Verification items for the finished model (mm, model axes). Face numbers are marked on the shaded views. A direction names the side the tool comes from. Coordinates: 2 decimals unless noted, no trailing zeros. Order: outer loops, then holes, each group sorted by start corner. A loop starts at its lowest first (then second) coordinate and runs counter-clockwise, first axis right, second up. Notation, with made-up numbers: M -35,6 L -1,6 A19 ccw -1,26 Z; hole C 89.5,29.25 d11. An arc over 180 degrees is marked long. Answer as a JSON object with one key per item and string values. Group by question number.
(1) Cross-section at C-C (y = -298). Enter the section's corners in (x, z).
(2) Cross-section at A-A (x = 70). Enter the section's corners in (y, z).
(3) Access from +Z, -Z, +X, -X, +Y, -Y to the whole of each face (thin tool, end or side, straight path). Record for the marked faces 1 and 2.
(4) Cross-section at B-B (z = 962). Enter the section's corners in (x, y), plus the area to 3 significant figures.
(5) Material ranges on line 1 (Y direction, x = 101, z = 986); line 2 (X direction, y = -295, z = 1023); line 3 (Z direction, x = 77.5, y = -305.5), recorded low to high.
(6) Cross-section at D-D (x = 33.5). Enter the section's corners in (y, z).
(7) Mould release check, pull along Y, two halves, no side actions. Record for the marked faces 3, 4 and 5: released by +Y, released by -Y, zero draft, split by the parting line, or undercut.
(8) Gauge pin test, flat ends, axial feed: pin 1 Ø2 at (y, z) = (-320, 1013.5) entering from -X; pin 2 Ø6 at (x, z) = (75, 963.5) entering from -Y; pin 3 Ø1 at (x, y) = (47.5, -287.5) entering from -Z. Record the tip position at first contact, or that the pin passes through.
from build123d import *

# Parameters (mm, degrees)
SKETCH1_R           = 45
SKETCH1_R_2         = 22.5
BOSS_EXTRUDE1_DEPTH = 30
SKETCH2_R           = 22.5
BOSS_EXTRUDE2_DEPTH = 60
FILLET1_R           = 10


with BuildPart() as part:
    # Sketch1 → Boss-Extrude1 (new body)
    with BuildSketch(Plane.XZ.offset(270)):
        with Locations((70, 999.189515243)):
            Circle(SKETCH1_R)
        with Locations((70, 999.189515243)):
            Circle(SKETCH1_R_2, mode=Mode.SUBTRACT)
    extrude(amount=BOSS_EXTRUDE1_DEPTH)

    # Sketch2 → Boss-Extrude2 (add)
    with BuildSketch(Plane.XZ.offset(270)):
        with Locations((70, 999.189515243)):
            Circle(SKETCH2_R)
    extrude(amount=BOSS_EXTRUDE2_DEPTH)

    # Fillet1
    fillet1_edges = [part.edges().sort_by_distance(p)[0] for p in [
        (47.5, -330, 999.189515243),
    ]]
    fillet(fillet1_edges, radius=FILLET1_R)


solid = part.part
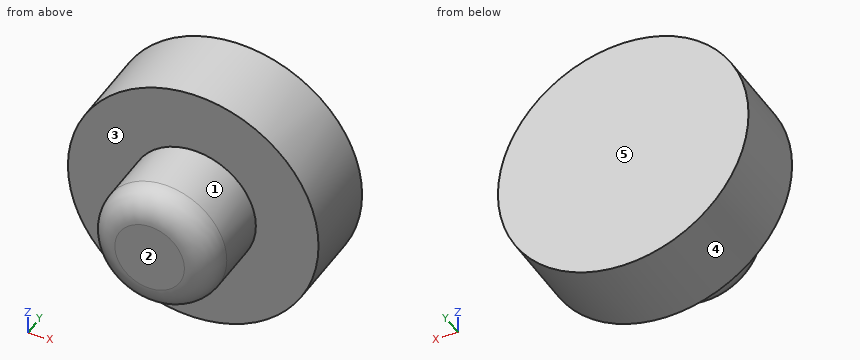
Taken from the geometry:
{
 "1": {"outline": "C 70,999.19 d90"},
 "2": {"outline": "M -330,986.69 A10 ccw -320,976.69 L -300,976.69 L -300,954.19 L -270,954.19 L -270,1044.19 L -300,1044.19 L -300,1021.69 L -320,1021.69 A10 ccw -330,1011.69 Z"},
 "3": {"face 1": "-Y", "face 2": "+Z, -Z, +X, -X, -Y"},
 "4": {"outline": "M 44.66,-300 L 95.34,-300 L 95.34,-270 L 44.66,-270 Z", "area": "1,520 mm²"},
 "5": {"line 1": "y = -300 to -270", "line 2": "x = 31.82 to 108.18", "line 3": "z = 977.98 to 1020.4"},
 "6": {"outline": "M -300,972.87 L -270,972.87 L -270,1025.51 L -300,1025.51 Z"},
 "7": {"face 3": "released by -Y", "face 4": "zero draft", "face 5": "released by +Y"},
 "8": {"pin 1": "stops at x = 51.86", "pin 2": "stops at y = -300", "pin 3": "stops at z = 959.93"}
}
